Input: part model. Units: mm. Frame: model coordinates. Face numbers are marked on the shaded views. Give positions to 0.01 mm unless a question says otherwise; leave off trailing zeros. Write each loop counter-clockwise with the first axis right and the second up, starting at its lowest first coordinate (ties: lowest second). Pieces come first, ordered by that corner, then holes. Notation, with made-up numbers: (87, 28.25) -> (111, 28.25) arc R22 cw to (111, 52.25) -> close; hole circle Ø3 at (1.25, 85.5). An arc over 180 degrees is marked (long way). Return JSON: item names as keys, results as strings. Group by question number.
Item 1: Section A-A, the plane z = 16. Count the separate pieces of the cut face and the enclosed holes in it, then the cut area to 3 significant figures.
Item 2: Section B-B, the plane x = 50. Return loops of the section in (y, z), then the cut area to 3 significant figures.
Item 3: Line query: line 1 (Y direction, x = -62, z = 8.5); line 2 (Y direction, x = 50, z = 7.5); line 3 (Y direction, x = 17, z = 6). Output: solid intervals per line, ascending. Write a range as [from, to].
Item 4: Section C-C, the plane y = -8. Return loops of the section in (x, z).
Item 5: Mould query, pull axis Y, two halves, no side actions, for the marked faces 1, 2, 3 and 4. Classes: released by +Y, released by -Y, zero draft, split by the parting line, or undercut.
Item 6: Section D-D, the plane x = -57. Return loops of the section in (y, z).
Item 7: Pin query (flat end, axial travel): P1, Ø3, axis at x = -50.5, z = 15.5, coming from the -Y side; P2, Ø3.5, axis at x = -62, y = 18, coming from the +Z side; P3, Ø1, axis at x = 32.5, y = -7.5, coming from the +Z side; P4, Ø1.2, axis at x = -50.5, z = 15.5, coming from the +Y side. Return the tip coordinate at first contact, or that it passes through.
from build123d import *

# Parameters (mm, degrees)
F0_W     = 50
F0_H     = 50
F0_R     = 2.5
F0_R_2   = 19
F0_W_2   = 40
F1_DEPTH = 12
F2_R     = 5
F3_W     = 15
F3_H     = 6
F3_W_2   = 10
F4_DEPTH = 6
F5_R     = 2.99999
F6_R     = 1.4
F7_DEPTH = 18


# Not quite as in the source:
# - a fillet or chamfer is up to 0.001 mm smaller than in the source, because OpenCascade refuses the exact size


with BuildPart() as f1:
    # F0 (on Top) → F1 (new body)
    with BuildSketch(Plane.XY):
        Rectangle(F0_W, F0_H)
        with Locations((-16.9705627485, -16.9705627485)):
            Circle(F0_R, mode=Mode.SUBTRACT)
        with Locations((16.9705627485, -16.9705627485)):
            Circle(F0_R, mode=Mode.SUBTRACT)
        with Locations((-16.9705627485, 16.9705627485)):
            Circle(F0_R, mode=Mode.SUBTRACT)
        Circle(F0_R_2, mode=Mode.SUBTRACT)
        with Locations((16.9705627485, 16.9705627485)):
            Circle(F0_R, mode=Mode.SUBTRACT)
        with Locations((45, 0)):
            Rectangle(F0_W_2, F0_H)
        with Locations((50, -15)):
            Circle(F0_R, mode=Mode.SUBTRACT)
        with Locations((50, 15)):
            Circle(F0_R, mode=Mode.SUBTRACT)
        with Locations((-50, 0)):
            Rectangle(F0_W, F0_H)
    extrude(amount=F1_DEPTH)

    # F2
    f2_edges = [f1.edges().sort_by_distance(p)[0] for p in [
        (65, -25, 6),
        (65, 25, 6),
        (-75, -25, 6),
        (-75, 25, 6),
    ]]
    fillet(f2_edges, radius=F2_R)

    # F3 (on face) → F4 (join)
    with BuildSketch(Plane.XY.offset(12)):
        with Locations((-47.5, 18)):
            Rectangle(F3_W, F3_H)
        with Locations((-60, 18)):
            Rectangle(F3_W_2, F3_H)
        with Locations((-47.5, -18)):
            Rectangle(F3_W, F3_H)
        with Locations((-60, -18)):
            Rectangle(F3_W_2, F3_H)
        Polygon((-46.5, 6.5), (-55, 6.5), (-55, 1.5), (-52, 1.5), (-52, 2.85), (-49.5, 2.85), (-49.5, 1.5), (-46.5, 1.5), align=None)
        Polygon((-46.5, -6.5), (-46.5, -1.5), (-49.5, -1.5), (-49.5, -2.85), (-52, -2.85), (-52, -1.5), (-55, -1.5), (-55, -6.5), align=None)
    extrude(amount=F4_DEPTH)

    # F5 (radius 3 in the source; OpenCascade refuses exactly that, so slightly less here)
    f5_edges = [f1.edges().sort_by_distance(p)[0] for p in [
        (-65, 21, 15),
        (-65, 15, 15),
        (-40, 15, 15),
        (-65, -15, 15),
        (-65, -21, 15),
        (-40, -21, 15),
        (-40, -15, 15),
        (-40, 21, 15),
    ]]
    fillet(f5_edges, radius=F5_R)

    # F6 (on face) → F7 (cut, through all)
    with BuildSketch(Plane.XY.offset(18)):
        with Locations((-62, 18)):
            Circle(F6_R)
        with Locations((-62, -18)):
            Circle(F6_R)
    extrude(amount=-F7_DEPTH, mode=Mode.SUBTRACT)


solid = f1.part
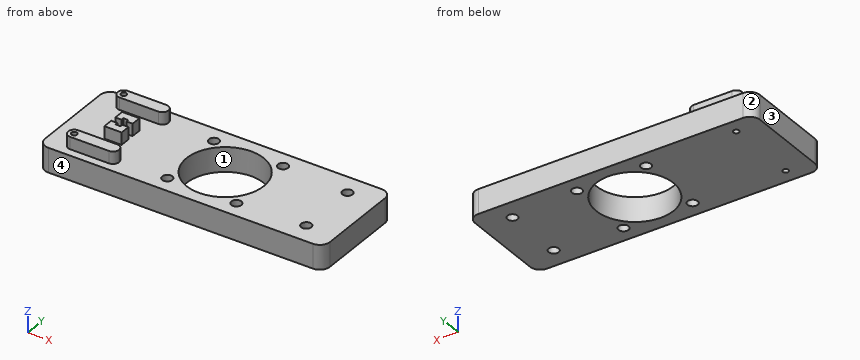
Answer below:
{
 "1": {"separate pieces": "4", "enclosed holes": "2", "area": "350 mm2"},
 "2": {"outline": "(-25, 0) -> (-17.5, 0) -> (-17.5, 12) -> (-25, 12) -> close; (-12.5, 0) -> (12.5, 0) -> (12.5, 12) -> (-12.5, 12) -> close; (17.5, 0) -> (25, 0) -> (25, 12) -> (17.5, 12) -> close", "area": "480 mm2"},
 "3": {"line 1": "y = [-25, -19.4], [-16.6, 16.6], [19.4, 25]", "line 2": "y = [-25, -17.5], [-12.5, 12.5], [17.5, 25]", "line 3": "y = [-25, -19.47], [-14.47, -8.49], [8.49, 14.47], [19.47, 25]"},
 "4": {"outline": "(-75, 0) -> (-17.23, 0) -> (-17.23, 12) -> (-75, 12) -> close; (17.23, 0) -> (65, 0) -> (65, 12) -> (17.23, 12) -> close"},
 "5": {"face 1": "undercut", "face 2": "released by +Y", "face 3": "zero draft", "face 4": "released by -Y"},
 "6": {"outline": "(-25, 0) -> (25, 0) -> (25, 12) -> (21, 12) -> (21, 18) -> (15, 18) -> (15, 12) -> (-15, 12) -> (-15, 18) -> (-21, 18) -> (-21, 12) -> (-25, 12) -> close"},
 "7": {"P1": "stops at y = -21", "P2": "stops at z = 18", "P3": "stops at z = 12", "P4": "stops at y = 21"}
}
